```python
from build123d import *

# Parameters (mm, degrees)
SKETCH1_W                           = 30
SKETCH1_H                           = 57.2
SKETCH1_W_2                         = 11.9888
SKETCH1_H_2                         = 11.9888
BOSS_EXTRUDE1_DEPTH                 = 10
SKETCH1_7_W                         = 11.9888
SKETCH1_7_H                         = 11.9888
SKETCH1_7_W_2                       = 8.9408
SKETCH1_7_H_2                       = 8.9408
BOSS_EXTRUDE2_DEPTH                 = 9
SKETCH1_8_W                         = 8.9408
SKETCH1_8_H                         = 8.9408
SKETCH1_8_R                         = 4
BOSS_EXTRUDE3_DEPTH                 = 11
F_4_40_TAPPED_HOLE1_D               = 2.2606
CUT_EXTRUDE1_START                  = 10
SKETCH3_R                           = 4.125
CUT_EXTRUDE1_DEPTH                  = 5.75
F_4_40_TAPPED_HOLE2_D               = 2.2606
F_4_40_TAPPED_HOLE2_DEPTH           = 7.59
F_4_40_TAPPED_HOLE2_TIP             = 0.679152758
F_4_40_TAPPED_HOLE2_ON_FACE_2_D     = 2.2606
F_4_40_TAPPED_HOLE2_ON_FACE_2_DEPTH = 7.59
F_4_40_TAPPED_HOLE2_ON_FACE_2_TIP   = 0.679152758
F_4_40_TAPPED_HOLE2_ON_FACE_3_D     = 2.2606
F_4_40_TAPPED_HOLE2_ON_FACE_3_DEPTH = 7.59
F_4_40_TAPPED_HOLE2_ON_FACE_3_TIP   = 0.679152758
F_4_40_TAPPED_HOLE2_ON_FACE_4_D     = 2.2606
F_4_40_TAPPED_HOLE2_ON_FACE_4_DEPTH = 7.59
F_4_40_TAPPED_HOLE2_ON_FACE_4_TIP   = 0.679152758


with BuildPart() as part:
    # Sketch1 → Boss-Extrude1 (new body)
    with BuildSketch(Plane.XY):
        with Locations((0, -9.5754)):
            Rectangle(SKETCH1_W, SKETCH1_H)
        Rectangle(SKETCH1_W_2, SKETCH1_H_2, mode=Mode.SUBTRACT)
    extrude(amount=BOSS_EXTRUDE1_DEPTH)

    # Sketch1<7> → Boss-Extrude2 (add)
    with BuildSketch(Plane.XY):
        Rectangle(SKETCH1_7_W, SKETCH1_7_H)
        Rectangle(SKETCH1_7_W_2, SKETCH1_7_H_2, mode=Mode.SUBTRACT)
    extrude(amount=BOSS_EXTRUDE2_DEPTH)

    # Sketch1<8> → Boss-Extrude3 (add)
    with BuildSketch(Plane.XY):
        Rectangle(SKETCH1_8_W, SKETCH1_8_H)
        Circle(SKETCH1_8_R, mode=Mode.SUBTRACT)
    extrude(amount=BOSS_EXTRUDE3_DEPTH)

    # #4-40 Tapped Hole1 (through all)
    with Locations(Plane(origin=(-7.5, 15.0246, 10), x_dir=(1, 0, 0), z_dir=(0, 0, 1))):
        with Locations((0, 0), (15, 0), (0, -30.2), (0, -40.2), (15, -30.2), (15, -40.2)):
            Hole(F_4_40_TAPPED_HOLE1_D / 2)

    # Sketch3 → Cut-Extrude1 (cut)
    with BuildSketch(Plane.XY.offset(CUT_EXTRUDE1_START)):
        with Locations((7.5, -15.1754)):
            Circle(SKETCH3_R)
        Polygon((4.325, -17.008487105), (4.325, -13.342312895), (7.5, -11.509225791), (10.675, -13.342312895), (10.675, -17.008487105), (7.5, -18.841574209), align=None, mode=Mode.SUBTRACT)
        Polygon((4.325, -13.342312895), (7.5, -11.509225791), (10.675, -13.342312895), (10.675, -17.008487105), (7.5, -18.841574209), (4.325, -17.008487105), align=None)
        with Locations((7.5, 15.0246)):
            Circle(SKETCH3_R)
        with Locations((-7.5, 15.0246)):
            Circle(SKETCH3_R)
        with Locations((-7.5, -15.1754)):
            Circle(SKETCH3_R)
    extrude(amount=-CUT_EXTRUDE1_DEPTH, mode=Mode.SUBTRACT)

    # #4-40 Tapped Hole2
    with Locations(Plane(origin=(9, -38.1754, 5), x_dir=(0, 0, -1), z_dir=(0, -1, 0))):
        with Locations((0, 0), (0, -18), (0, -14), (0, -4)):
            Hole(F_4_40_TAPPED_HOLE2_D / 2, depth=F_4_40_TAPPED_HOLE2_DEPTH)
            with Locations((0, 0, -(F_4_40_TAPPED_HOLE2_DEPTH + F_4_40_TAPPED_HOLE2_TIP / 2))):  # 118° drill point
                Cone(0, F_4_40_TAPPED_HOLE2_D / 2, F_4_40_TAPPED_HOLE2_TIP, mode=Mode.SUBTRACT)

    # #4-40 Tapped Hole2 on face 2
    with Locations(Plane(origin=(0, 19.0246, 5), x_dir=(0, 0, 1), z_dir=(0, 1, 0))):
        with Locations((0, 0)):
            Hole(F_4_40_TAPPED_HOLE2_ON_FACE_2_D / 2, depth=F_4_40_TAPPED_HOLE2_ON_FACE_2_DEPTH)
            with Locations((0, 0, -(F_4_40_TAPPED_HOLE2_ON_FACE_2_DEPTH + F_4_40_TAPPED_HOLE2_ON_FACE_2_TIP / 2))):  # 118° drill point
                Cone(0, F_4_40_TAPPED_HOLE2_ON_FACE_2_D / 2, F_4_40_TAPPED_HOLE2_ON_FACE_2_TIP, mode=Mode.SUBTRACT)

    # #4-40 Tapped Hole2 on face 3
    with Locations(Plane(origin=(15, 6.3546, 4), x_dir=(0, 0, 1), z_dir=(1, 0, 0))):
        with Locations((0, 0), (0, 12.7)):
            Hole(F_4_40_TAPPED_HOLE2_ON_FACE_3_D / 2, depth=F_4_40_TAPPED_HOLE2_ON_FACE_3_DEPTH)
            with Locations((0, 0, -(F_4_40_TAPPED_HOLE2_ON_FACE_3_DEPTH + F_4_40_TAPPED_HOLE2_ON_FACE_3_TIP / 2))):  # 118° drill point
                Cone(0, F_4_40_TAPPED_HOLE2_ON_FACE_3_D / 2, F_4_40_TAPPED_HOLE2_ON_FACE_3_TIP, mode=Mode.SUBTRACT)

    # #4-40 Tapped Hole2 on face 4
    with Locations(Plane(origin=(-15, 6.3546, 4), x_dir=(0, 0, -1), z_dir=(-1, 0, 0))):
        with Locations((0, 0), (0, 12.7)):
            Hole(F_4_40_TAPPED_HOLE2_ON_FACE_4_D / 2, depth=F_4_40_TAPPED_HOLE2_ON_FACE_4_DEPTH)
            with Locations((0, 0, -(F_4_40_TAPPED_HOLE2_ON_FACE_4_DEPTH + F_4_40_TAPPED_HOLE2_ON_FACE_4_TIP / 2))):  # 118° drill point
                Cone(0, F_4_40_TAPPED_HOLE2_ON_FACE_4_D / 2, F_4_40_TAPPED_HOLE2_ON_FACE_4_TIP, mode=Mode.SUBTRACT)


solid = part.part
```
Geometry check sheet. Reference: the model listing, model coordinates, mm. A direction names the side the tool comes from. Round coordinates to 2 decimals unless told otherwise and drop trailing zeros. Loops run counter-clockwise (first coordinate to the right, second up) from the corner with the lowest first, then second, coordinate; pieces in that order, holes last. Notation, with made-up numbers: (4, 45) -> (13, 45) arc R23 ccw to (13, 60) -> close; hole circle Ø11 at (44.25, 38). An arc over 180 degrees is marked (long way). Use a Markdown table: item, result.
(1) Sectioned sample at B-B (z = 1.75). Enter the section's corners in (x, y), then the cut area to 3 significant figures.
Calculated:
| item | result |
|---|---|
| outline | (-15, -38.18) -> (15, -38.18) -> (15, 19.02) -> (-15, 19.02) -> close; hole circle Ø2.26 at (-7.5, -25.18); hole circle Ø2.26 at (-7.5, -15.18); hole circle Ø2.26 at (-7.5, 15.02); hole circle Ø8 at (0, 0); hole circle Ø2.26 at (7.5, -25.18); hole circle Ø2.26 at (7.5, -15.18); hole circle Ø2.26 at (7.5, 15.02) |
| area | 1,640 mm² |
(2) Scan lines: probe 1 along Y at (x, z) = (7.5, 2.7); probe 2 along X at (y, z) = (-35.75, 5); probe 3 along Y at (x, z) = (-7.5, 5.9). Record each from-to range of solid material in increasing order.
Calculated:
| item | result |
|---|---|
| probe 1 | -38.18 to -26.31, -24.05 to -16.31, -14.05 to 13.89, 16.15 to 19.02 |
| probe 2 | -15 to -10.13, -7.87 to -6.13, -3.87 to 3.87, 6.13 to 7.87, 10.13 to 15 |
| probe 3 | -38.18 to -26.31, -24.05 to -19.3, -11.05 to 10.9 |
(3) Set-up check for faces 3 (the cylindrical face through (6.892, 15.978, 2.095)), 4 (the flat face through (-0.1, 5.994, 9.5)), 5 (the cylindrical face through (9.34, -34.33, 6.08)), 6 (the cylindrical face through (-11.152, 7.458, 3.755)): record each of +Z, -Z, +X, -X, +Y, -Y from which the full face is reachable in a straight line by a thin tool's end or side.
Calculated:
| item | result |
|---|---|
| face 3 | +Z, -Z |
| face 4 | +Z |
| face 5 | -Y |
| face 6 | -X |
(4) Sectioned sample at C-C (y = 13). Enter the section's corners in (x, z).
Calculated:
| item | result |
|---|---|
| outline | (-15, 0) -> (15, 0) -> (15, 10) -> (11.09, 10) -> (11.09, 4.25) -> (3.91, 4.25) -> (3.91, 10) -> (-3.91, 10) -> (-3.91, 4.25) -> (-11.09, 4.25) -> (-11.09, 10) -> (-15, 10) -> close; hole circle Ø2.26 at (0, 5) |
(5) Go/stop test with flat-tipped pins: P1, Ø2.5, axis at x = -6, y = -13, coming from the +Z side; P2, Ø1.8, axis at y = 6.35, z = 4, coming from the +X side; P3, Ø1.4, axis at y = -6.35, z = 4, coming from the +X side; P4, Ø1.6, axis at x = 2, z = 10.5, coming from the +Y side. Record where each tip stops, or that it passes through.
Calculated:
| item | result |
|---|---|
| P1 | z = 4.25 |
| P2 | x = 7.27 |
| P3 | x = 7.15 |
| P4 | y = 19.02 |
(6) Mould release check, pull along Y, two halves, no side actions. Record for faces 1 (the flat face through (15, -10, 5)), 2 (the flat face through (-0.1, -5.994, 9.5)): released by +Y, released by -Y, zero draft, split by the parting line, or undercut.
Calculated:
| item | result |
|---|---|
| face 1 | zero draft |
| face 2 | undercut |
(7) Sectioned sample at A-A (x = -2). Enter the section's corners in (y, z), then the cut area to 3 significant figures.
Calculated:
| item | result |
|---|---|
| outline | (-38.18, 0) -> (-3.46, 0) -> (-3.46, 11) -> (-4.47, 11) -> (-4.47, 9) -> (-5.99, 9) -> (-5.99, 10) -> (-38.18, 10) -> close; (3.46, 0) -> (19.02, 0) -> (19.02, 10) -> (5.99, 10) -> (5.99, 9) -> (4.47, 9) -> (4.47, 11) -> (3.46, 11) -> close |
| area | 502 mm² |
